Study the drawing (mm; zero at the part's minimum x, y, z) and answer. Give positions to 0.01 mm unless a question says otherwise; leave off trailing zeros. Write each loop counter-clockwise with the first axis right and the second up, starting at its lowest first coordinate (ties: lowest second). Pieces come first, ordered by that corner, then holes. Notation, with made-up numbers: (-40, -9.5) - (-34, -9.5) arc R22 ccw to (-34, 14.5) - close; hole circle Ø9 at (18, 20). An arc over 180 degrees is marked (long way). Answer as CSV lines item,"result".
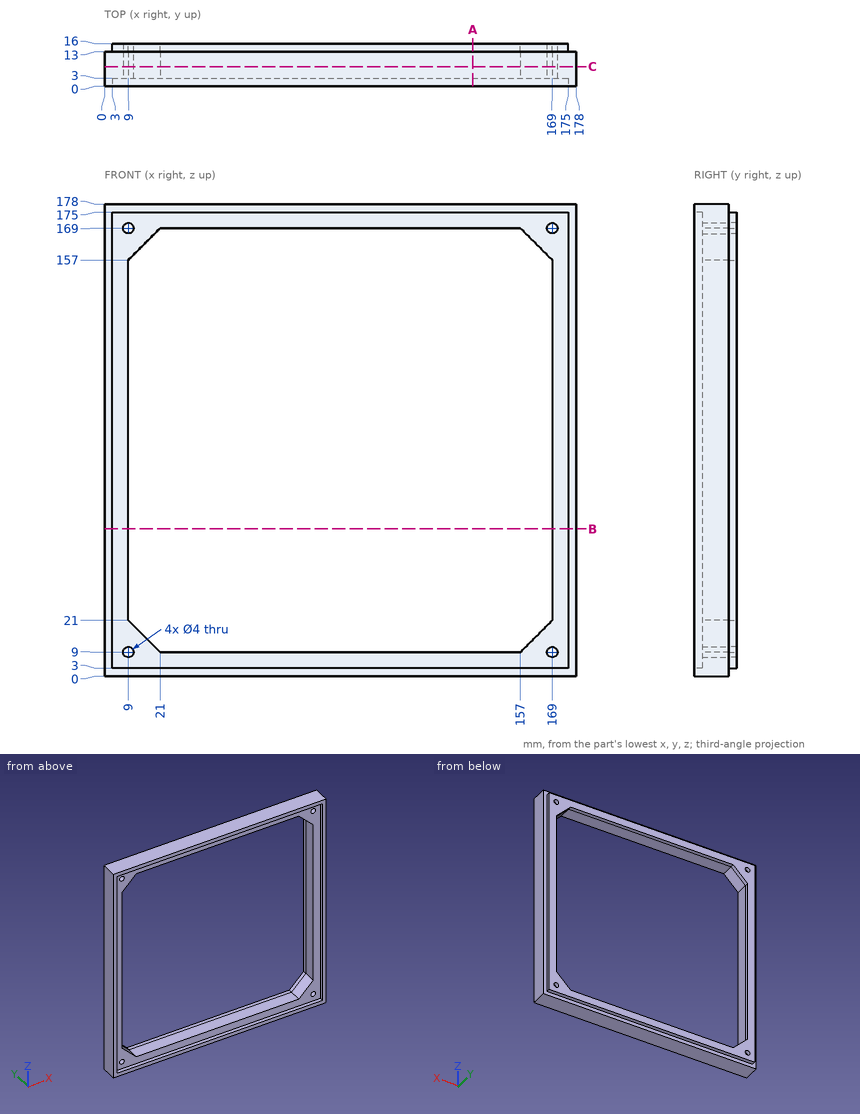
(1) A cutting plane is placed at A-A (x = 139). Write down the section's boundary in (y, z).
Worked out:
outline,"(0, 0) - (13, 0) - (13, 3) - (16, 3) - (16, 9) - (3, 9) - (3, 3) - (0, 3) - close; (0, 175) - (3, 175) - (3, 169) - (16, 169) - (16, 175) - (13, 175) - (13, 178) - (0, 178) - close"
(2) A cutting plane is placed at B-B (z = 55.5). Write down the section's boundary in (x, y), and give its area (3 significant figures).
Worked out:
outline,"(0, 0) - (3, 0) - (3, 3) - (9, 3) - (9, 16) - (3, 16) - (3, 13) - (0, 13) - close; (169, 3) - (175, 3) - (175, 0) - (178, 0) - (178, 13) - (175, 13) - (175, 16) - (169, 16) - close"
area,"234 mm^2"
(3) Find the intervals of material crossed by L1, parallel to Z at x = 79, y = 14.5; L2, parallel to Z at x = 152, y = 2; L3, parallel to X at y = 12.25, z = 111, in increasing order.
Worked out:
L1,"z = 3 to 9, 169 to 175"
L2,"z = 0 to 3, 175 to 178"
L3,"x = 0 to 9, 169 to 178"
(4) A cutting plane is placed at C-C (y = 7.5). Write down the section's boundary in (x, z), and give its area (3 significant figures).
Worked out:
outline,"(0, 0) - (178, 0) - (178, 178) - (0, 178) - close; hole circle Ø4 at (9, 9); hole circle Ø4 at (9, 169); hole (9, 21) - (21, 9) - (157, 9) - (169, 21) - (169, 157) - (157, 169) - (21, 169) - (9, 157) - close; hole circle Ø4 at (169, 9); hole circle Ø4 at (169, 169)"
area,"6,320 mm^2"
(5) Each of these flat-tipped pins is pushed along its axis until it touches: P1, Ø6.5, axis at x = 9, z = 169, coming from the -Y side; P2, Ø0.9, axis at x = 106.5, y = 14.5, coming from the +Z side; P3, Ø1.5, axis at y = 15, z = 67.5, coming from the +X side. Where does it stop, or does it pass through?
Worked out:
P1,"stops at y = 3"
P2,"stops at z = 175"
P3,"stops at x = 175"
